Study the drawing (mm; zero at the part's minimum x, y, z) and answer. A direction names the side the tool comes from. Coordinates: 2 decimals unless noted, no trailing zeros. Loops run counter-clockwise (first coordinate to the right, second up) from the corner with the lowest first, then second, coordinate; pieces in that order, holes last. Notation, with made-up numbers: (50.5, 44.25) - (66.5, 44.25) arc R17 ccw to (66.5, 69.25) - close; hole circle Ø6 at (49.5, -6.75). An arc over 180 degrees is marked (long way). Use CSV: the item, a comma, the result in double quotes.
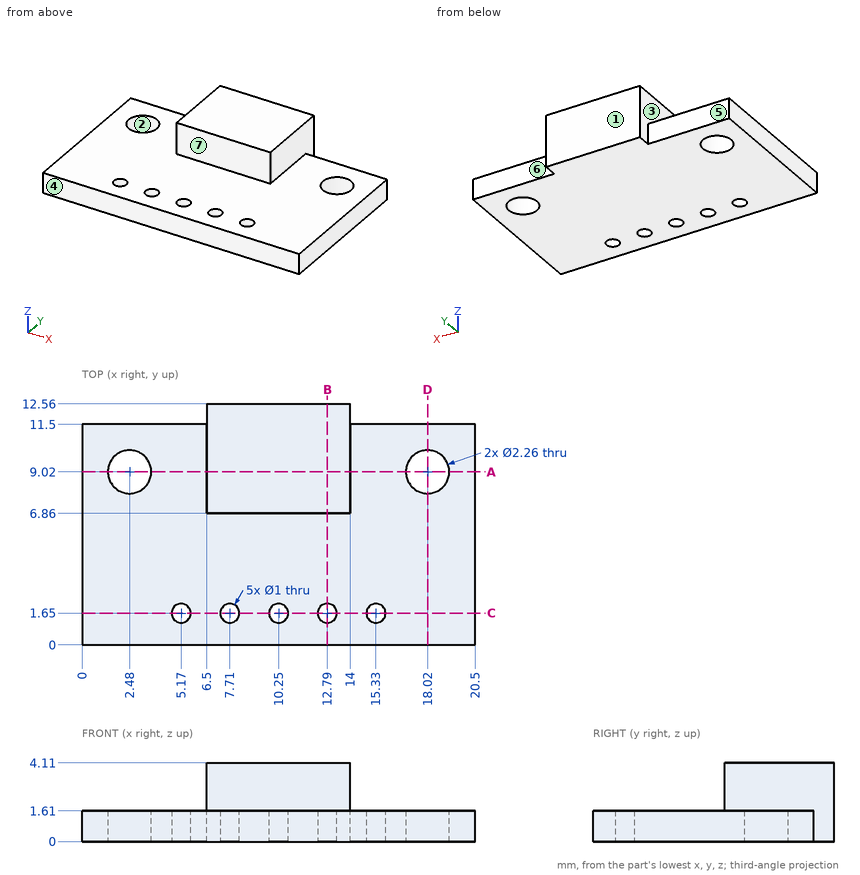
Q1. The part is cut by section A-A on y = 9.02. Determine the outline of the cut face in (x, z), and give its area (3 significant figures).
Reported:
outline,"(0, 0) - (1.35, 0) - (1.35, 1.61) - (0, 1.61) - close; (3.61, 0) - (16.89, 0) - (16.89, 1.61) - (14, 1.61) - (14, 4.11) - (6.5, 4.11) - (6.5, 1.61) - (3.61, 1.61) - close; (19.15, 0) - (20.5, 0) - (20.5, 1.61) - (19.15, 1.61) - close"
area,"44.5 mm²"
Q2. The part is cut by section D-D on x = 18.02. Determine the outline of the cut face in (y, z).
Reported:
outline,"(0, 0) - (7.89, 0) - (7.89, 1.61) - (0, 1.61) - close; (10.15, 0) - (11.5, 0) - (11.5, 1.61) - (10.15, 1.61) - close"
Q3. For a pull along Y with two mould halves and no side action, classify the marked faces 1, 2, 3 and 4 as +Y half, -Y half, draft (parallel to the pull), parting line (faces both ways), or undercut.
Reported:
face 1,"+Y half"
face 2,"undercut"
face 3,"draft"
face 4,"-Y half"
Q4. The part is cut by section C-C on y = 1.65. Determine the outline of the cut face in (x, z).
Reported:
outline,"(0, 0) - (4.67, 0) - (4.67, 1.61) - (0, 1.61) - close; (5.67, 0) - (7.21, 0) - (7.21, 1.61) - (5.67, 1.61) - close; (8.21, 0) - (9.75, 0) - (9.75, 1.61) - (8.21, 1.61) - close; (10.75, 0) - (12.29, 0) - (12.29, 1.61) - (10.75, 1.61) - close; (13.29, 0) - (14.83, 0) - (14.83, 1.61) - (13.29, 1.61) - close; (15.83, 0) - (20.5, 0) - (20.5, 1.61) - (15.83, 1.61) - close"
Q5. The part is cut by section B-B on x = 12.79. Determine the outline of the cut face in (y, z).
Reported:
outline,"(0, 0) - (1.15, 0) - (1.15, 1.61) - (0, 1.61) - close; (2.15, 0) - (12.56, 0) - (12.56, 4.11) - (6.86, 4.11) - (6.86, 1.61) - (2.15, 1.61) - close"
Q6. Find the intervals of material crossed by probe 1 along X at (y, z) = (9.25, 0.5); probe 2 along Y at (x, z) = (12.79, 0.4); probe 3 along Y at (x, z) = (15.33, 0.8), in increasing order. Write a range as [from, to].
Reported:
probe 1,"x = [0, 1.37], [3.59, 16.91], [19.13, 20.5]"
probe 2,"y = [0, 1.15], [2.15, 12.56]"
probe 3,"y = [0, 1.15], [2.15, 11.5]"
Q7. Given P1, Ø1.4, axis at x = 18.02, y = 9.02, coming from the -Z side; P2, Ø2, axis at x = 3, y = 9, coming from the -Z side; P3, Ø1.3, axis at x = 4.5, z = 1, coming from the +Y side; P4, Ø4, axis at x = 11.5, y = 4.5, coming from the +Z side, each flat-ended and moving along its own axis, determine where each tip first touches the part or whether it passes through.
Reported:
P1,"passes through"
P2,"stops at z = 0"
P3,"stops at y = 11.5"
P4,"stops at z = 1.61"
Q8. A tool of negligible diameter and unlimited length cuts with its end or side. For the marked faces 5, 6 and 7, from which of +Z, -Z, +X, -X, +Y, -Y can it reach the whole face along a straight path? Write none if from no direction.
Reported:
face 5,"+Z, -Z, -X, +Y"
face 6,"+Z, -Z, +X, +Y"
face 7,"+Z, +X, -X, -Y"
